```python
from build123d import *

# Parameters (mm, degrees)
CUT_EXTRUDE1_DEPTH = 2.38125
FILLET1_R          = 0.396875
FILLET2_R          = 0.79375
CHAMFER1_SIZE      = 0.254


with BuildPart() as part:
    # Sketch1 → Revolve1 (revolve)
    with BuildSketch(Plane.XY):
        Polygon((1.5875, 0), (4.7625, 0), (4.7625, 3.96875), (2.921, 3.96875), (2.921, 13.49375), (1.5875, 13.49375), align=None)
    revolve(axis=Axis((0, 7.886499903, 0), (0, -1, 0)))

    # Sketch2 → Cut-Extrude1 (cut)
    with BuildSketch(Plane.XZ):
        Polygon((1.75976362, 3.048), (-1.75976362, 3.048), (-3.519527241, 0), (-1.75976362, -3.048), (1.75976362, -3.048), (3.519527241, 0), align=None)
    extrude(amount=-CUT_EXTRUDE1_DEPTH, mode=Mode.SUBTRACT)

    # Fillet1
    fillet1_edges = [part.edges().sort_by_distance(p)[0] for p in [
        (-2.921, 3.96875, 0),
    ]]
    fillet(fillet1_edges, radius=FILLET1_R)

    # Fillet2
    fillet2_edges = [part.edges().sort_by_distance(p)[0] for p in [
        (2.639645431, 2.38125, 1.524),
        (1.75976362, 1.190625, 3.048),
        (2.639645431, 2.38125, -1.524),
        (3.519527241, 1.190625, 0),
        (0, 2.38125, -3.048),
        (1.75976362, 1.190625, -3.048),
        (-2.639645431, 2.38125, -1.524),
        (-1.75976362, 1.190625, -3.048),
        (-2.639645431, 2.38125, 1.524),
        (-3.519527241, 1.190625, 0),
        (0, 2.38125, 3.048),
        (-1.75976362, 1.190625, 3.048),
    ]]
    fillet(fillet2_edges, radius=FILLET2_R)

    # Chamfer1
    chamfer1_edges = [part.edges().sort_by_distance(p)[0] for p in [
        (-1.5875, 2.38125, 0),
        (2.639645431, 0, -1.524),
        (0, 0, -3.048),
        (-2.639645431, 0, -1.524),
        (-2.639645431, 0, 1.524),
        (-1.5875, 13.49375, 0),
        (2.639645431, 0, 1.524),
        (-2.921, 13.49375, 0),
        (0, 0, 3.048),
        (3.396733689, 0, 0),
        (1.698366844, 0, -2.941657664),
        (-1.698366844, 0, -2.941657664),
        (-3.396733689, 0, 0),
        (1.698366844, 0, 2.941657664),
        (-1.698366844, 0, 2.941657664),
        (-4.7625, 3.96875, 0),
        (-4.7625, 0, 0),
    ]]
    chamfer(chamfer1_edges, length=CHAMFER1_SIZE)


solid = part.part
```
Geometry check sheet. Reference: the model listing, model coordinates, mm. A direction names the side the tool comes from. Round coordinates to 2 decimals unless told otherwise and drop trailing zeros. Write each loop counter-clockwise with the first axis right and the second up, starting at its lowest first coordinate (ties: lowest second). Pieces come first, ordered by that corner, then holes. Notation, with made-up numbers: (39.25, 34.5) - (78.25, 34.5) arc R13 ccw to (78.25, 55.5) - close; hole circle Ø6 at (26, -5). An arc over 180 degrees is marked (long way). Write each question's results on one line, items separated by ' | '.
(1) Thickness scan on probe 1 along Z at (x, y) = (0, 11); probe 2 along Y at (x, z) = (-3.5, 2.75); probe 3 along Z at (x, y) = (0.75, 11.25). Record the ranges inside material, lowest first. Write a range as from..to.
Computed:
probe 1: z = -2.92..-1.59, 1.59..2.92 | probe 2: y = 0..3.97 | probe 3: z = -2.82..-1.4, 1.4..2.82
(2) Draft check along X on faces 1 (the face through (2, 3.969, 3)), 2 (the face through (-0.633, 8.865, -2.852)), 3 (the face through (0, 2.381, 2)). Enter one of: pulls with the +X half, pulls with the -X half, needs draft (parallel to the pull), parting line crosses it, or undercut.
Computed:
face 1: needs draft | face 2: parting line crosses it | face 3: undercut
(3) Depth check by flat-ended pin: pin 1 Ø5 at (x, y) = (0.5, 10) entering from -Z; pin 2 Ø5 at (x, z) = (0, 0) entering from -Y. Enter the tip coordinate at first touch or a pass-through.
Computed:
pin 1: stops at z = -2.92 | pin 2: stops at y = 2.34
(4) Sectioned sample at B-B, the plane y = 11.5. Enter the section's corners in (x, z) (1 decimal), plus the area to 3 significant figures.
Computed:
outline: circle Ø5.8 at (0, 0); hole circle Ø3.2 at (0, 0) | area: 18.9 mm^2
(5) Set-up check for faces 4 (the face through (-2.65, 0.91, -1.51)), 5 (the face through (-3.78, 2.01, -2.9)): record each of +Z, -Z, +X, -X, +Y, -Y from which the full face is reachable in a straight line by a thin tool's end or side.
Computed:
face 4: -Y | face 5: +Y, -Y
